For this review, use the dimensioned drawing (mm, ordinates from the lowest corner) and the shaded views. A direction names the side the tool comes from. Coordinates: 2 decimals unless noted, no trailing zeros. Order: outer loops, then holes, each group sorted by start corner. A loop starts at its lowest first (then second) coordinate and runs counter-clockwise, first axis right, second up. Notation, with made-up numbers: (24.25, -3) -> (39.25, -3) arc R14 cw to (39.25, 17) -> close; hole circle Ø1 at (40.5, 58.25). An arc over 180 degrees is marked (long way). Use one line per item in the form item = value. Start each with the question number.
(1) Take a section at C-C (y = 19.5). State the section outline as (x, z) points.
(2) Take a section at D-D (y = 37.5). State the section outline as (x, z) points (1 decimal).
(3) Take a section at A-A (z = 9). State the section outline as (x, y) points, then the cut area to 4 significant figures.
(4) Wall thickness on line 1 along Y through (x, z) = (24, 40) (1 decimal); line 2 along X through (y, z) = (21, 10); line 3 along Y through (x, z) = (26, 12): over which ranges is each line inside the solid? List them lowest first.
(5) For the marked faces 4 and 5, list the 3-axis set-ups (+Z, -Z, +X, -X, +Y, -Y) from which the entire face can be reached by the end or side of a thin tool; tool diameter is ignored.
(6) Mouldability with a two-part tool opening along X and no side actions: class the marked faces 1, 2 and 3 as +X half, -X half, draft (parallel to the pull), parting line (faces both ways), or undercut.
(7) Take a section at B-B (x = 21.5). State the section outline as (y, z) points (1 decimal).
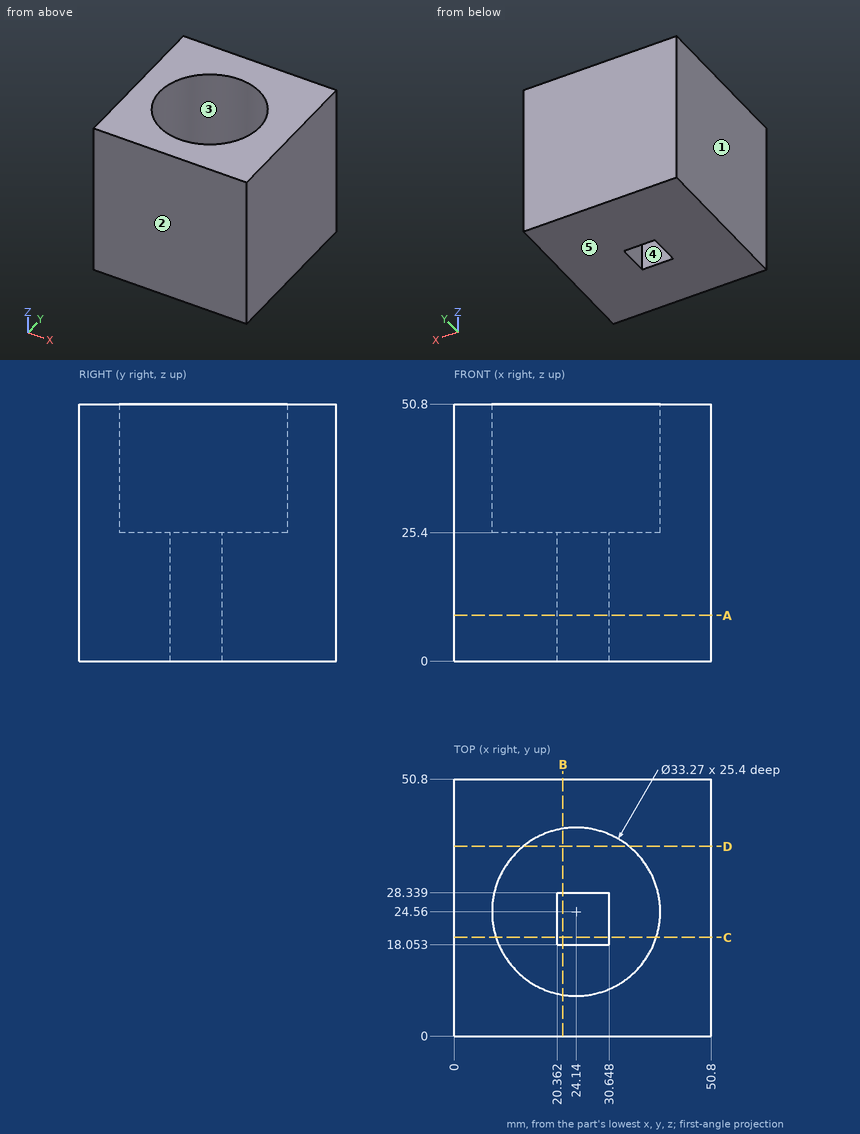
Findings:
q1.outline = (0, 0) -> (20.36, 0) -> (20.36, 25.4) -> (8.29, 25.4) -> (8.29, 50.8) -> (0, 50.8) -> close; (30.65, 0) -> (50.8, 0) -> (50.8, 50.8) -> (39.99, 50.8) -> (39.99, 25.4) -> (30.65, 25.4) -> close
q2.outline = (0, 0) -> (50.8, 0) -> (50.8, 50.8) -> (34.6, 50.8) -> (34.6, 25.4) -> (13.7, 25.4) -> (13.7, 50.8) -> (0, 50.8) -> close
q3.outline = (0, 0) -> (50.8, 0) -> (50.8, 50.8) -> (0, 50.8) -> close; hole (20.36, 18.05) -> (30.65, 18.05) -> (30.65, 28.34) -> (20.36, 28.34) -> close
q3.area = 2,475 mm²
q4.line_1 = 0 to 7.9, 41.2 to 50.8
q4.line_2 = 0 to 20.36, 30.65 to 50.8
q4.line_3 = 0 to 18.05, 28.34 to 50.8
q5.face_4 = +Z, -Z
q5.face_5 = -Z, +X, -X, +Y, -Y
q6.face_1 = -X half
q6.face_2 = draft
q6.face_3 = undercut
q7.outline = (0, 0) -> (18.1, 0) -> (18.1, 25.4) -> (8.1, 25.4) -> (8.1, 50.8) -> (0, 50.8) -> close; (28.3, 0) -> (50.8, 0) -> (50.8, 50.8) -> (41, 50.8) -> (41, 25.4) -> (28.3, 25.4) -> close
